Design review of the part built by this model. Coordinates are the model's own, in mm. A direction names the side the tool comes from. Give positions to 0.01 mm unless a question says otherwise; leave off trailing zeros. Loops run counter-clockwise (first coordinate to the right, second up) from the corner with the lowest first, then second, coordinate; pieces in that order, holes last. Notation, with made-up numbers: (-22.75, -22.75) - (23.25, -22.75) arc R18 ccw to (23.25, 2.25) - close; hole circle Ø7 at (32.25, -1). An arc over 180 degrees is marked (long way). Write each question's results on one line, items separated by ' | '.
from build123d import *

# Parameters (mm, degrees)
SKETCH_1_R      = 7.1
SKETCH_1_R_2    = 3
EXTRUDE_1_DEPTH = 5
SKETCH_1_3_R    = 7.1
SKETCH_1_3_R_2  = 2.1
EXTRUDE_2_DEPTH = 3
FILLET_1_R      = 1
FILLET_2_R      = 1
FILLET_3_R      = 1
FILLET_4_R      = 1


with BuildPart() as part:
    # Sketch 1 → Extrude 1 (new body)
    with BuildSketch(Plane(origin=(0, 0, 0), x_dir=(1, 0, 0), z_dir=(0, 1, 0))):
        with BuildLine():
            Line((1.92, -15.884382267), (51.2, -9.927738917))
            ThreePointArc((51.2, -9.927738917), (60, 0), (51.2, 9.927738917))
            Line((51.2, 9.927738917), (1.92, 15.884382267))
            ThreePointArc((1.92, 15.884382267), (-16, 0), (1.92, -15.884382267))
        make_face()
        with Locations(Location((50, 0, 0), (0, 0, 270))):
            Circle(SKETCH_1_R, mode=Mode.SUBTRACT)
        with Locations(Location((0, 0, 0), (0, 0, 270))):
            Circle(SKETCH_1_R_2, mode=Mode.SUBTRACT)
        Polygon((18.356508588, 8.861251331), (38.535462938, 6.422151611), (30.734984007, 2.266153232), align=None, mode=Mode.SUBTRACT)
        Polygon((18.356508588, -8.861251331), (38.535462938, -6.422151611), (30.734984007, -2.266153232), align=None, mode=Mode.SUBTRACT)
        with BuildLine():
            Line((14.72234722, 6.265180949), (26.481594346, 0))
            Line((26.481594346, 0), (14.72234722, -6.265180949))
            ThreePointArc((14.72234722, -6.265180949), (16, 0), (14.72234722, 6.265180949))
        make_face(mode=Mode.SUBTRACT)
        with BuildLine():
            Line((34.988373668, 0), (40.429404433, -2.898913674))
            ThreePointArc((40.429404433, -2.898913674), (40, 0), (40.429404433, 2.898913674))
            Line((40.429404433, 2.898913674), (34.988373668, 0))
        make_face(mode=Mode.SUBTRACT)
    extrude(amount=EXTRUDE_1_DEPTH)

    # Sketch 1_3 → Extrude 2 (add)
    with BuildSketch(Plane(origin=(0, 0, 0), x_dir=(1, 0, 0), z_dir=(0, 1, 0))):
        with Locations(Location((50, 0, 0), (0, 0, 270))):
            Circle(SKETCH_1_3_R)
        with Locations(Location((50, 0, 0), (0, 0, 270))):
            Circle(SKETCH_1_3_R_2, mode=Mode.SUBTRACT)
    extrude(amount=EXTRUDE_2_DEPTH)

    # Fillet 1
    fillet_1_edges = [part.edges().sort_by_distance(p)[0] for p in [
        (34.988373668, 2.5, 0),
        (40.429404433, 2.5, 2.898913674),
        (40.429404433, 2.5, -2.898913674),
    ]]
    fillet(fillet_1_edges, radius=FILLET_1_R)

    # Fillet 2
    fillet_2_edges = [part.edges().sort_by_distance(p)[0] for p in [
        (18.356508588, 2.5, 8.861251331),
        (38.535462938, 2.5, 6.422151611),
        (30.734984007, 2.5, 2.266153232),
    ]]
    fillet(fillet_2_edges, radius=FILLET_2_R)

    # Fillet 3
    fillet_3_edges = [part.edges().sort_by_distance(p)[0] for p in [
        (38.535462938, 2.5, -6.422151611),
        (18.356508588, 2.5, -8.861251331),
        (30.734984007, 2.5, -2.266153232),
    ]]
    fillet(fillet_3_edges, radius=FILLET_3_R)

    # Fillet 4
    fillet_4_edges = [part.edges().sort_by_distance(p)[0] for p in [
        (26.481594346, 2.5, 0),
        (14.72234722, 2.5, -6.265180949),
        (14.72234722, 2.5, 6.265180949),
    ]]
    fillet(fillet_4_edges, radius=FILLET_4_R)


solid = part.part
(1) Draft analysis for pull direction Z (two halves, no side actions). For faces 3 (the cylindrical face through (60, 2, 0)), 4 (the flat face through (37.625, 2.465, -1.405)), 5 (the cylindrical face through (15.843, 2.535, -4.976)), state which applies: pulls with the +Z half, pulls with the -Z half, needs draft (parallel to the pull), parting line crosses it, or undercut.
Answers below:
face 3: parting line crosses it | face 4: undercut | face 5: undercut
(2) Take a section at D-D on x = 28.5. Give the boundary of the cut face in (y, z), plus the area to 3 significant figures.
Answers below:
outline: (0, -12.67) - (5, -12.67) - (5, -7.64) - (0, -7.64) - close; (0, -3.46) - (5, -3.46) - (5, 3.46) - (0, 3.46) - close; (0, 7.64) - (5, 7.64) - (5, 12.67) - (0, 12.67) - close | area: 84.9 mm2
(3) Take a section at B-B on x = 0. Give the boundary of the cut face in (y, z).
Answers below:
outline: (0, -16) - (5, -16) - (5, -3) - (0, -3) - close; (0, 3) - (5, 3) - (5, 16) - (0, 16) - close
(4) Take a section at A-A on y = 1.25. Count the separate pieces of the cut face and the enclosed holes in it, plus the area to 3 significant figures.
Answers below:
separate pieces: 1 | enclosed holes: 6 | area: 1,660 mm2
(5) Take a section at C-C on z = 0. Give the boundary of the cut face in (x, y).
Answers below:
outline: (-16, 0) - (-3, 0) - (-3, 5) - (-16, 5) - close; (3, 0) - (16, 0) - (16, 5) - (3, 5) - close; (25.35, 0) - (36.12, 0) - (36.12, 5) - (25.35, 5) - close; (40, 0) - (47.9, 0) - (47.9, 3) - (42.9, 3) - (42.9, 5) - (40, 5) - close; (52.1, 0) - (60, 0) - (60, 5) - (57.1, 5) - (57.1, 3) - (52.1, 3) - close
(6) Tool access review of faces 1 (the flat face through (26.724, 2.465, -4.403)), 2 (the flat face through (48.5, 3, -1.7)): name each direction out of +Z, -Z, +X, -X, +Y, -Y from which nothing blocks a thin tool from reaching the whole face with its end or side.
Answers below:
face 1: +Y, -Y | face 2: +Y
(7) Wall thickness on line 1 along X through (y, z) = (3.7, 0); line 2 along X through (y, z) = (1.55, 0); line 3 along X through (y, z) = (3.7, 6.5): over which ranges is each line inside the solid? List them lowest first. Write a range as from..to.
Answers below:
line 1: -16..-3, 3..16, 25.35..36.12, 40..42.9, 57.1..60 | line 2: -16..-3, 3..16, 25.35..36.12, 40..47.9, 52.1..60 | line 3: -14.62..22.86, 35.99..47.14, 52.86..57.6
